from build123d import *

# Parameters (mm, degrees)
BOSS_EXTRUDE1_DEPTH = 50
CHAMFER2_SIZE       = 1
CHAMFER3_SIZE       = 4


with BuildPart() as part:
    # Sketch1 → Boss-Extrude1 (new body)
    with BuildSketch(Plane.XY):
        Polygon((0, 0), (-20, 0), (-20, -60), (-25, -60), (-25, 5), (-21, 5), (-21, 30), (-11, 30), (-11, 25), (-16, 25), (-16, 19), (-11, 19), (-11, 17.5), (0, 17.5), (0, 14), (-16, 14), (-16, 5), (0, 5), align=None)
    boss_extrude1 = extrude(amount=BOSS_EXTRUDE1_DEPTH)

    # Mirror1: Boss-Extrude1 across plane
    add(boss_extrude1.mirror(Plane(origin=(0, 5, 50), x_dir=(0, 0, 1), z_dir=(-1, 0, 0))))

    # Chamfer2
    chamfer2_edges = [part.edges().sort_by_distance(p)[0] for p in [
        (-16, 30, 0),
        (-11, 27.5, 0),
        (-13.5, 25, 0),
        (-16, 22, 0),
        (-13.5, 19, 0),
        (-11, 30, 25),
        (-11, 25, 25),
        (-11, 19, 25),
        (-13.5, 19, 50),
        (-16, 22, 50),
        (-13.5, 25, 50),
        (-11, 27.5, 50),
        (-16, 30, 50),
        (16, 30, 50),
        (11, 27.5, 50),
        (11, 30, 25),
        (13.5, 25, 50),
        (11, 25, 25),
        (16, 22, 50),
        (13.5, 19, 50),
        (11, 19, 25),
        (13.5, 19, 0),
        (16, 22, 0),
        (13.5, 25, 0),
        (11, 27.5, 0),
        (16, 30, 0),
    ]]
    chamfer(chamfer2_edges, length=CHAMFER2_SIZE)

    # Chamfer3
    chamfer3_edges = [part.edges().sort_by_distance(p)[0] for p in [
        (21, 5, 25),
        (-21, 5, 25),
    ]]
    chamfer(chamfer3_edges, length=CHAMFER3_SIZE - 0.0001)  # a hair under: the kernel refuses the full size


solid = part.part
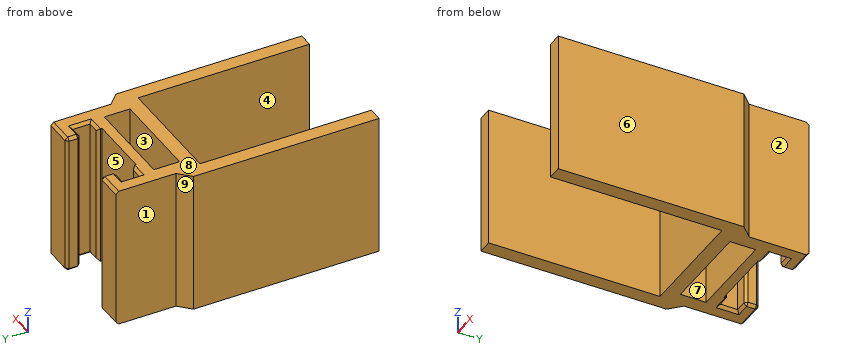
Read the model definition and answer for the solid it produces. Units are mm, in the model's axes. Face numbers are marked on the shaded views. A direction names the side the tool comes from. Give positions to 0.01 mm unless a question says otherwise; leave off trailing zeros. Write each loop counter-clockwise with the first axis right and the second up, starting at its lowest first coordinate (ties: lowest second). Pieces come first, ordered by that corner, then holes. Notation, with made-up numbers: M 80.25,-38 L 118.25,-38 A26 cw 118.25,-18 Z; hole C 66.5,-31.75 d3. An arc over 180 degrees is marked long. One line per item, written item: value. Start each with the question number.
(1) Find section B-B (x = -2.5). Determine the outline of the cut face in (y, z).
(2) Find section A-A (y = -38). Determine the outline of the cut face in (x, z), plus the area to 3 significant figures.
(3) Find the intervals of material crossed by line 1 (X direction, y = -37, z = 25); line 2 (Y direction, x = 1.5, z = 16.5); line 3 (Y direction, x = 17, z = 25), in increasing order.
(4) A tool of negligible diameter and unlimited length cuts with its end or side. For the marked faces 1, 2, 3, 4 and 5, from which of +Z, -Z, +X, -X, +Y, -Y can it reach the whole face along a straight path? Write none if from no direction.
(5) Find section C-C (x = -13). Determine the outline of the cut face in (y, z), plus the area to 3 significant figures.
(6) Determine the mould class of the marked faces 6, 7, 8 and 9 for opening direction X: pulls with the +X half, pulls with the -X half, needs draft (parallel to the pull), parting line crosses it, or undercut.
(7) Flat-ended cylindrical pins translate along their axes: pin 1 Ø10 at (y, z) = (11, 37) entering from -X; pin 2 Ø17.5 at (x, z) = (3.5, 36) entering from +Y; pin 3 Ø6.5 at (y, z) = (21, 25) entering from -X; pin 4 Ø2 at (x, z) = (13.5, 19) entering from -Y. Find the tip coordinate at first contact, or state that the pin passes through.
Results below:
1. outline: M 0,0 L 5,0 L 5,50 L 0,50 Z; M 14,0 L 17.5,0 L 17.5,50 L 14,50 Z
2. outline: M -25,0 L -20,0 L -20,50 L -25,50 Z; M 20,0 L 25,0 L 25,50 L 20,50 Z
2. area: 500 mm^2
3. line 1: x = -25 to -20, 20 to 25
3. line 2: y = 0 to 5, 14 to 17.5
3. line 3: y = 0 to 30
4. face 1: +Z, -Z, -X, +Y
4. face 2: +Z, -Z, +X, +Y
4. face 3: +Z, -Z
4. face 4: +Z, -Z, -Y
4. face 5: +Z, -Z, +Y
5. outline: M 0,0 L 5,0 L 5,50 L 0,50 Z; M 14,0 L 18,0 L 19,1 L 19,49 L 18,50 L 14,50 Z; M 25,1 L 26,0 L 29,0 L 30,1 L 30,49 L 29,50 L 26,50 L 25,49 Z
5. area: 747 mm^2
6. face 6: pulls with the +X half
6. face 7: undercut
6. face 8: needs draft
6. face 9: pulls with the -X half
7. pin 1: stops at x = -24
7. pin 2: stops at y = 30
7. pin 3: stops at x = -21
7. pin 4: stops at y = 0
